from build123d import *

# Parameters (mm, degrees)
SKETCH_W        = 55
SKETCH_H        = 56
PAD_DEPTH       = 18
SKETCH012_W     = 52.6
SKETCH012_H     = 53.6
POCKET_DEPTH    = 16.8
POCKET001_DEPTH = 1.2
SKETCH014_W     = 19.5
SKETCH014_H     = 7.5
POCKET002_DEPTH = 1.2
SKETCH015_R     = 2.5
SKETCH015_R_2   = 0.9
PAD010_DEPTH    = 2.5


with BuildPart() as part:
    # Sketch → Pad (new body)
    with BuildSketch(Plane.XY):
        Rectangle(SKETCH_W, SKETCH_H)
    extrude(amount=PAD_DEPTH)

    # Sketch012 (on Face6 of Pad) → Pocket (cut)
    with BuildSketch(Plane.XY.offset(18)):
        Rectangle(SKETCH012_W, SKETCH012_H)
    extrude(amount=-POCKET_DEPTH, mode=Mode.SUBTRACT)

    # Sketch013 (on Face6 of Pocket) → Pocket001 (cut)
    with BuildSketch(Plane.XZ.offset(28)):
        with BuildLine():
            ThreePointArc((12.47, 9.000073), (15.239982, 11.74), (12.49, 14.5))
            Line((9.66, 14.5), (12.49, 14.5))
            Line((9.66, 14.5), (9.962666, 15.767791))
            ThreePointArc((9.962666, 15.767791), (9.774923, 16.619593), (8.99, 17))
            Line((-9.01, 17), (8.99, 17))
            ThreePointArc((-9.01, 17), (-9.794923, 16.619593), (-9.982666, 15.767791))
            Line((-9.68, 14.5), (-9.982666, 15.767791))
            Line((-12.51, 14.5), (-9.68, 14.5))
            ThreePointArc((-12.51, 14.5), (-15.26, 11.75), (-12.51, 9))
            Line((-12.51, 9), (-8.39, 9))
            Line((-7.983449, 7.271094), (-8.39, 9))
            ThreePointArc((-7.983449, 7.271094), (-7.630924, 6.716129), (-7.01, 6.5))
            Line((6.99, 6.5), (-7.01, 6.5))
            ThreePointArc((6.99, 6.5), (7.615236, 6.719564), (7.965913, 7.281839))
            Line((7.965913, 7.281839), (8.35, 9))
            Line((8.35, 9), (12.47, 9.000073))
        make_face()
    extrude(amount=-POCKET001_DEPTH, mode=Mode.SUBTRACT)

    # Sketch014 (on Face2 of Pocket001) → Pocket002 (cut)
    with BuildSketch(Plane(origin=(-27.5, 0, 0), x_dir=(0, -1, 0), z_dir=(-1, 0, 0))):
        with Locations((2.75, 8.25)):
            Rectangle(SKETCH014_W, SKETCH014_H)
    extrude(amount=-POCKET002_DEPTH, mode=Mode.SUBTRACT)

    # Sketch015 (on Face31 of Pocket002) → Pad010 (join)
    with BuildSketch(Plane.XY.offset(1.2)):
        with Locations((22, -23.05)):
            Circle(SKETCH015_R)
        with Locations((22, -23.05)):
            Circle(SKETCH015_R_2, mode=Mode.SUBTRACT)
        with Locations((-22, -23.05)):
            Circle(SKETCH015_R)
        with Locations((-22, -23.05)):
            Circle(SKETCH015_R_2, mode=Mode.SUBTRACT)
        with Locations((22, 20.95)):
            Circle(SKETCH015_R)
        with Locations((22, 20.95)):
            Circle(SKETCH015_R_2, mode=Mode.SUBTRACT)
        with Locations((-22, 20.95)):
            Circle(SKETCH015_R)
        with Locations((-22, 20.95)):
            Circle(SKETCH015_R_2, mode=Mode.SUBTRACT)
    extrude(amount=PAD010_DEPTH)


solid = part.part
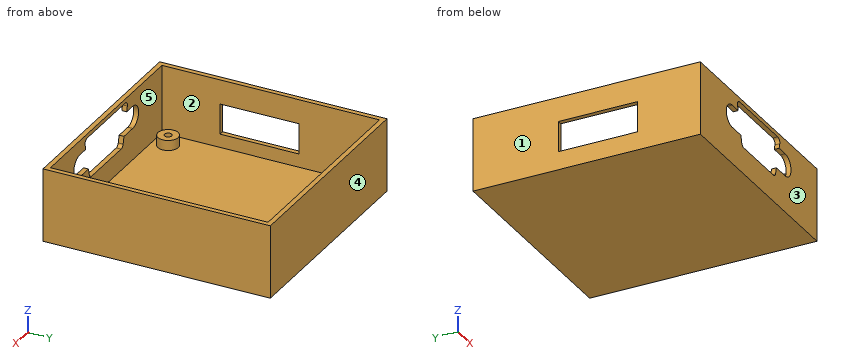
Here's how the part is built. I have some questions about the finished solid (model axes, mm). Face numbers are marked on the shaded views. A direction names the side the tool comes from. Round coordinates to 2 decimals unless told otherwise and drop trailing zeros. Loops run counter-clockwise (first coordinate to the right, second up) from the corner with the lowest first, then second, coordinate; pieces in that order, holes last. Notation, with made-up numbers: (82, 24.25) - (135, 24.25) arc R9 cw to (135, 29.25) - close; hole circle Ø2 at (28.25, -11.5). An arc over 180 degrees is marked (long way). One line per question, with ' | ' between items. Start each with the question number.
Q1. For the marked faces 4 and 5, which set-ups out of +Z, -Z, +X, -X, +Y, -Y let a thin tool reach every point of the face, with its end or its side?
Q2. I want a section at B-B (y = 6). Write out the boundary of the cut face in (x, z).
Q3. Will these pins go through, and if not, where does the flat tip stop? pin 1 (1.5 mm diameter, centred on x = -21, y = 22, fed in from +Z); pin 2 (0.5 mm diameter, centred on x = -22, y = 21, fed in from +Z).
Q4. I want a section at C-C (x = 3.5). Write out the boundary of the cut face in (y, z).
Q5. We'd pull the mould along X, two halves only. Please class the marked faces 1, 2 and 3: +X half, -X half, draft (parallel to the pull), parting line (faces both ways), or undercut.
Q6. I want a section at A-A (z = 2.5). State how many separate pieces and enclosed holes the cut face has, then the cut area to 3 significant figures.
Q7. I want a section at D-D (y = 16). Write out the boundary of the cut face in (x, z), then the cut area to 3 significant figures.
Q8. Please list where these lines run through material, in increasing order: line 1 (Y direction, x = -22, z = 2.7); line 2 (X direction, y = -13, z = 7); line 3 (Y direction, x = -19, z = 2). Write a range as [from, to].
Response values:
1) face 4: +Z, -Z, +X, -X, +Y | face 5: +Z
2) outline: (-27.5, 0) - (27.5, 0) - (27.5, 18) - (26.3, 18) - (26.3, 1.2) - (-26.3, 1.2) - (-26.3, 4.5) - (-27.5, 4.5) - close; (-27.5, 12) - (-26.3, 12) - (-26.3, 18) - (-27.5, 18) - close
3) pin 1: stops at z = 3.7 | pin 2: stops at z = 1.2
4) outline: (-28, 0) - (28, 0) - (28, 18) - (26.8, 18) - (26.8, 1.2) - (-26.8, 1.2) - (-26.8, 6.5) - (-28, 6.5) - close; (-28, 17) - (-26.8, 17) - (-26.8, 18) - (-28, 18) - close
5) face 1: -X half | face 2: undercut | face 3: draft
6) separate pieces: 5 | enclosed holes: 5 | area: 329 mm²
7) outline: (-27.5, 0) - (27.5, 0) - (27.5, 18) - (26.3, 18) - (26.3, 1.2) - (-26.3, 1.2) - (-26.3, 18) - (-27.5, 18) - close | area: 106 mm²
8) line 1: y = [-28, -26.8], [-25.55, -23.95], [-22.15, -20.55], [18.45, 20.05], [21.85, 23.45], [26.8, 28] | line 2: x = [-27.5, -26.3], [26.3, 27.5] | line 3: y = [-28, -26.8], [26.8, 28]
